The listing builds one solid part. Answer for the finished solid, in the listing's coordinates (mm). A direction names the side the tool comes from. Round coordinates to 2 decimals unless told otherwise and drop trailing zeros. Loops run counter-clockwise (first coordinate to the right, second up) from the corner with the lowest first, then second, coordinate; pieces in that order, holes last. Notation, with made-up numbers: (79, 33.5) - (115, 33.5) arc R19 cw to (115, 39.5) - close; hole circle Ø6 at (52.5, 81). An arc over 180 degrees is marked (long way). Write item = value, one per line. Start each with the question number.
1) Section A-A, the plane x = -17 is taken. Determine the outline of the cut face in (y, z) (3 decimals), and give its area (3 significant figures).
2) For a pull along Y with two mould halves and no side action, classify faces 3 (the cylindrical face through (15.277, -1.576, 1.035)), 4 (the flat face through (-11.4, 47.5, 8.3)), 5 (the flat face through (38, -1, 11)), 6 (the cylindrical face through (35.3, 37.28, 1.04)) as released by +Y, released by -Y, zero draft, split by the parting line, or undercut.
3) Straight lines are drawn through the part: line 1 along X through (y, z) = (35.75, 1.65) (3 decimals); line 2 along X through (y, z) = (-35.5, 0.95) (3 decimals); line 3 along Y through (x, z) = (34.5, 1.1) (3 decimals). For each, find the intervals that lie inside material, in ascending order.
4) Section D-D, the plane x = -29.5 is taken. Determine the outline of the cut face in (y, z), and give its area (4 significant figures).
5) Given pin 1 Ø5 at (x, y) = (-11, 18.5) entering from -Z; pin 2 Ø3 at (x, y) = (8, 5.5) entering from +Z; pin 3 Ø3 at (x, y) = (34.5, -35.75) entering from +Z, each flat-ended and moving along its own axis, determine where each tip first touches the part or whether it passes through.
6) Section B-B, the plane z = 5.5 is taken. Give the number of separate pieces and of enclosed holes in the cut face, and give its area (4 significant figures).
7) A tool of negligible diameter and unlimited length cuts with its end or side. For faces 1 (the flat face through (8, -1, 2.1)), 2 (the cylindrical face through (16.626, -33.816, 1.035)), from which of +Z, -Z, +X, -X, +Y, -Y can it reach the whole face along a straight path? Write none if from no direction.
from build123d import *

# Parameters (mm, degrees)
F0_W     = 76
F0_H     = 95
F1_DEPTH = 21.4
F2_W     = 8
F2_H     = 19.3
F2_W_2   = 6.428571
F2_W_3   = 6.428572
F3_DEPTH = 95
F4_R     = 1.725
F5_DEPTH = 2.1


with BuildPart() as f1:
    # F0 (on Top) → F1 (new body)
    with BuildSketch(Plane.XY):
        Rectangle(F0_W, F0_H)
    extrude(amount=F1_DEPTH)

    # F2 (on face) → F3 (cut, through all)
    with BuildSketch(Plane.XZ.offset(47.5)):
        with Locations((-32.5, 11.75)):
            Rectangle(F2_W, F2_H)
        with Locations((32.5, 11.75)):
            Rectangle(F2_W, F2_H)
        with Locations((-23.785714, 11.75)):
            Rectangle(F2_W_2, F2_H)
        with Locations((-15.857143, 11.75)):
            Rectangle(F2_W_3, F2_H)
        with Locations((-7.928571, 11.75)):
            Rectangle(F2_W_2, F2_H)
        with Locations((0, 11.75)):
            Rectangle(F2_W_3, F2_H)
        with Locations((7.928571, 11.75)):
            Rectangle(F2_W_2, F2_H)
        with Locations((15.857143, 11.75)):
            Rectangle(F2_W_3, F2_H)
        with Locations((23.785714, 11.75)):
            Rectangle(F2_W_2, F2_H)
    extrude(amount=-F3_DEPTH, mode=Mode.SUBTRACT)

    # F4 (on face) → F5 (cut, through all)
    with BuildSketch(Plane(origin=(0, 0, 0), x_dir=(1, 0, 0), z_dir=(0, 0, -1))):
        with Locations((-17, 35.5)):
            Circle(F4_R)
        with Locations((17, 35.5)):
            Circle(F4_R)
        with Locations((17, 1.5)):
            Circle(F4_R)
        with Locations((-17, 1.5)):
            Circle(F4_R)
        with Locations((-34.5, 35.75)):
            Circle(F4_R)
        with Locations((34.5, 35.75)):
            Circle(F4_R)
        with Locations((34.5, -35.75)):
            Circle(F4_R)
        with Locations((-34.5, -35.75)):
            Circle(F4_R)
    extrude(amount=-F5_DEPTH, mode=Mode.SUBTRACT)


solid = f1.part
Geometry check:
q1.outline = (-47.5, 0) - (-37.225, 0) - (-37.225, 2.1) - (-47.5, 2.1) - close; (-33.775, 0) - (-3.225, 0) - (-3.225, 2.1) - (-33.775, 2.1) - close; (0.225, 0) - (47.5, 0) - (47.5, 2.1) - (0.225, 2.1) - close
q1.area = 185 mm2
q2.face_3 = undercut
q2.face_4 = released by +Y
q2.face_5 = zero draft
q2.face_6 = undercut
q3.line_1 = -38 to -36.225, -32.775 to 32.775, 36.225 to 38
q3.line_2 = -38 to -36.207, -32.793 to -18.725, -15.275 to 15.275, 18.725 to 32.793, 36.207 to 38
q3.line_3 = -47.5 to -37.475, -34.025 to 34.025, 37.475 to 47.5
q4.outline = (-47.5, 0) - (47.5, 0) - (47.5, 2.1) - (-47.5, 2.1) - close
q4.area = 199.5 mm2
q5.pin_1 = 0
q5.pin_2 = 2.1
q5.pin_3 = through
q6.separate_pieces = 10
q6.enclosed_holes = 0
q6.area = 1,425 mm2
q7.face_1 = +Z, +Y, -Y
q7.face_2 = +Z, -Z
